from build123d import *

# Parameters (mm, degrees)
SKETCH1_W           = 30
SKETCH1_H           = 30
BOSS_EXTRUDE1_DEPTH = 2
SKETCH2_R           = 1
SKETCH2_W           = 5
SKETCH2_H           = 2
CUT_EXTRUDE1_DEPTH  = 2
FILLET2_R           = 2


with BuildPart() as part:
    # Sketch1 → Boss-Extrude1 (new body)
    with BuildSketch(Plane(origin=(0, 0, 0), x_dir=(1, 0, 0), z_dir=(0, 1, 0))):
        Rectangle(SKETCH1_W, SKETCH1_H)
    extrude(amount=BOSS_EXTRUDE1_DEPTH)

    # Sketch2 → Cut-Extrude1 (cut)
    with BuildSketch(Plane(origin=(0, 2, 0), x_dir=(1, 0, 0), z_dir=(0, 1, 0))):
        with Locations(Location((10, 10, 0), (0, 0, 270))):
            Circle(SKETCH2_R)
        with Locations(Location((10, -10, 0), (0, 0, 90))):
            Circle(SKETCH2_R)
        with Locations(Location((-10, -10, 0), (0, 0, 270))):
            Circle(SKETCH2_R)
        with Locations(Location((-10, 10, 0), (0, 0, 90))):
            Circle(SKETCH2_R)
        with Locations((-2.5, 0)):
            Rectangle(SKETCH2_W, SKETCH2_H)
        with Locations((-10.5, 0)):
            Rectangle(SKETCH2_W, SKETCH2_H)
    extrude(amount=-CUT_EXTRUDE1_DEPTH, mode=Mode.SUBTRACT)

    # Fillet2
    fillet2_edges = [part.edges().sort_by_distance(p)[0] for p in [
        (-15, 1, -15),
        (15, 1, -15),
        (15, 1, 15),
        (-15, 1, 15),
    ]]
    fillet(fillet2_edges, radius=FILLET2_R)


solid = part.part
The listing builds one solid part. Answer for the finished solid, in the listing's coordinates (mm). A direction names the side the tool comes from. Give positions to 0.01 mm unless a question says otherwise; leave off trailing zeros. Loops run counter-clockwise (first coordinate to the right, second up) from the corner with the lowest first, then second, coordinate; pieces in that order, holes last. Notation, with made-up numbers: (-24.75, -12) - (33.25, -12) arc R19 ccw to (33.25, 25) - close; hole circle Ø8 at (-25.5, 44). An arc over 180 degrees is marked (long way). Use one line per item in the form item = value.
1. Given pin 1 Ø3 at (x, z) = (10, 10) entering from +Y; pin 2 Ø1.8 at (x, z) = (-10, -10) entering from +Y, each flat-ended and moving along its own axis, determine where each tip first touches the part or whether it passes through.
Calculated:
pin_1 = 2
pin_2 = through
2. Section B-B on z = -10 is taken. Give the vertices of the cut face in (x, y), then the cut area to 3 significant figures.
Calculated:
outline = (-15, 0) - (-11, 0) - (-11, 2) - (-15, 2) - close; (-9, 0) - (9, 0) - (9, 2) - (-9, 2) - close; (11, 0) - (15, 0) - (15, 2) - (11, 2) - close
area = 52.0 mm^2
3. Find the intervals of material crossed by line 1 along X through (y, z) = (1.05, 10); line 2 along X through (y, z) = (1.2, 0); line 3 along Z through (x, y) = (-9.75, 0.65), in increasing order. Write a range as [from, to].
Calculated:
line_1 = [-15, -11], [-9, 9], [11, 15]
line_2 = [-15, -13], [-8, -5], [0, 15]
line_3 = [-15, -10.97], [-9.03, -1], [1, 9.03], [10.97, 15]
4. Section D-D on y = 1.05 is taken. Give the vertices of the cut face in (x, z), then the cut area to 3 significant figures.
Calculated:
outline = (-15, -13) arc R2 ccw to (-13, -15) - (13, -15) arc R2 ccw to (15, -13) - (15, 13) arc R2 ccw to (13, 15) - (-13, 15) arc R2 ccw to (-15, 13) - close; hole (-13, -1) - (-8, -1) - (-8, 1) - (-13, 1) - close; hole circle Ø2 at (-10, -10); hole circle Ø2 at (-10, 10); hole (-5, -1) - (0, -1) - (0, 1) - (-5, 1) - close; hole circle Ø2 at (10, -10); hole circle Ø2 at (10, 10)
area = 864 mm^2
5. The mould has two halves that part along Z. Classify faces 3 (the face through (-15, 1, 0)), 4 (the face through (-5, 1, 0)), 5 (the face through (14.4, 1.01, -14.43)): pulls with the +Z half, pulls with the -Z half, needs draft (parallel to the pull), parting line crosses it, or undercut.
Calculated:
face_3 = needs draft
face_4 = undercut
face_5 = pulls with the -Z half
6. Section A-A on x = -10 is taken. Give the vertices of the cut face in (y, z), then the cut area to 3 significant figures.
Calculated:
outline = (0, -15) - (2, -15) - (2, -11) - (0, -11) - close; (0, -9) - (2, -9) - (2, -1) - (0, -1) - close; (0, 1) - (2, 1) - (2, 9) - (0, 9) - close; (0, 11) - (2, 11) - (2, 15) - (0, 15) - close
area = 48.0 mm^2
7. Section C-C on x = -0.75 is taken. Give the vertices of the cut face in (y, z), then the cut area to 3 significant figures.
Calculated:
outline = (0, -15) - (2, -15) - (2, -1) - (0, -1) - close; (0, 1) - (2, 1) - (2, 15) - (0, 15) - close
area = 56.0 mm^2
8. Which of the six approach directions +Z, -Z, +X, -X, +Y, -Y give full straight-line access (tool end or side, diameter ignored) to faces 1 (the face through (-11, 1, -1)), 2 (the face through (-14.43, 1.01, 14.4))?
Calculated:
face_1 = +Y, -Y
face_2 = +Z, -X, +Y, -Y
